from build123d import *

# Parameters (mm, degrees)
CROQUIS1_R              = 4
SALIENTE_EXTRUIR1_DEPTH = 3


with BuildPart() as part:
    # Croquis1 → Saliente-Extruir1 (new body)
    with BuildSketch(Plane(origin=(0, 0, 0), x_dir=(0, 0, -1), z_dir=(1, 0, 0))):
        Polygon((8, 0), (4, 6.92820323), (-4, 6.92820323), (-8, 0), (-4, -6.92820323), (4, -6.92820323), align=None)
        Circle(CROQUIS1_R, mode=Mode.SUBTRACT)
    extrude(amount=SALIENTE_EXTRUIR1_DEPTH)


solid = part.part
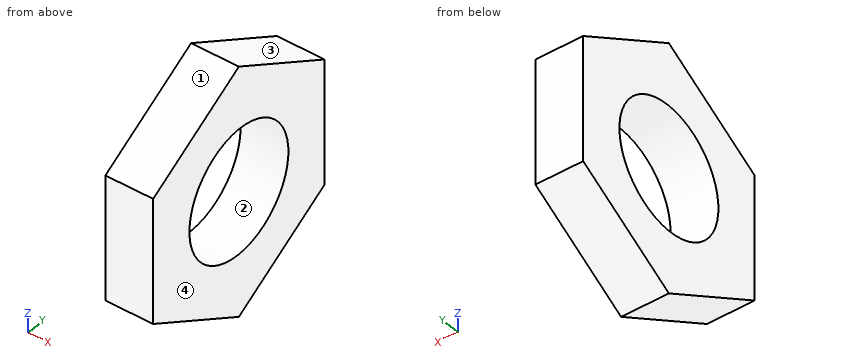
Build history of the part. All positions in model axes, mm. Face numbers are marked on the shaded views. Round coordinates to 2 decimals unless told otherwise and drop trailing zeros. Write each loop counter-clockwise with the first axis right and the second up, starting at its lowest first coordinate (ties: lowest second). Pieces come first, ordered by that corner, then holes. Notation, with made-up numbers: M -1,53.25 L 52,53.25 A29 ccw 52,79.25 Z; hole C 39.5,-7 d8. An arc over 180 degrees is marked long. Answer in a Markdown table with one row per item.
1. Saw through at D-D (z = -7). List the corners of the cut face in (x, y).
Geometry check:
| item | result |
|---|---|
| outline | M 0,-1.73 L 3,-1.73 L 3,1.73 L 0,1.73 Z |
2. Mould opens along Y. For the marked faces 1, 2, 3 and 4 say: +Y half, -Y half, draft (parallel to the pull), parting line (faces both ways), or undercut.
Geometry check:
| item | result |
|---|---|
| face 1 | -Y half |
| face 2 | undercut |
| face 3 | +Y half |
| face 4 | draft |
3. Saw through at A-A (z = 0). List the corners of the cut face in (x, y), and give its area (3 significant figures).
Geometry check:
| item | result |
|---|---|
| outline | M 0,-6.93 L 3,-6.93 L 3,-4 L 0,-4 Z; M 0,4 L 3,4 L 3,6.93 L 0,6.93 Z |
| area | 17.6 mm2 |
4. Probe L1, parallel to Y at x = 2.25, z = 0; L2, parallel to Z at x = 1.95, y = -2; L3, parallel to Y at x = 1.15, z = -1.5. List the from-to ranges inside material, lowest first. Write a range as [from, to].
Geometry check:
| item | result |
|---|---|
| L1 | [-6.93, -4], [4, 6.93] |
| L2 | [-6.85, -3.46], [3.46, 6.85] |
| L3 | [-6.93, -3.71], [3.71, 6.93] |
5. Saw through at C-C (x = 0.6). List the corners of the cut face in (y, z).
Geometry check:
| item | result |
|---|---|
| outline | M -6.93,-4 L 0,-8 L 6.93,-4 L 6.93,4 L 0,8 L -6.93,4 Z; hole C 0,0 d8 |
6. Saw through at B-B (y = 1.5). List the corners of the cut face in (x, z).
Geometry check:
| item | result |
|---|---|
| outline | M 0,-7.13 L 3,-7.13 L 3,-3.71 L 0,-3.71 Z; M 0,3.71 L 3,3.71 L 3,7.13 L 0,7.13 Z |
7. Flat gauge pins, fed straight in: P1, Ø7, axis at y = 0, z = 0, coming from the +X side; P2, Ø1.5, axis at y = -2.5, z = 5, coming from the -X side. Where does each tip first touch, or does it go through?
Geometry check:
| item | result |
|---|---|
| P1 | through |
| P2 | x = 0 |
